Read the model definition and answer for the solid it produces. Units are mm, in the model's axes. Give positions to 0.01 mm unless a question says otherwise; leave off trailing zeros. Order: outer loops, then holes, each group sorted by start corner. A loop starts at its lowest first (then second) coordinate and runs counter-clockwise, first axis right, second up. Notation, with made-up numbers: (22.25, -35.5) - (44.25, -35.5) arc R29 ccw to (44.25, -10.5) - close; hole circle Ø6 at (19.5, -20). An arc over 180 degrees is marked (long way). Use a Markdown table: item, result. Add a question column.
1. A flat-ended cylindrical pin translates along its axis: P1, Ø8.5, axis at x = 24, y = 15, coming from the +Z side. Find the tip coordinate at first contact, or state that the pin passes through.
2. For a pull along Y with two mould halves and no side action, classify faces 1 (the flat face through (109, 0, 5)), 2 (the cylindrical face through (109.1, 170.9, 4.9)), 3 (the flat face through (220, 175, 5)) as released by +Y, released by -Y, zero draft, split by the parting line, or undercut.
3. A cutting plane is placed at A-A on x = 110. Determine the outline of the cut face in (y, z).
4. Consider L1, parallel to Y at x = 24, z = 2.75; L2, parallel to Y at x = 109.5, z = 9.25; L3, parallel to X at y = 189.5, z = 1.75. Determine where each line is inside the solid, lowest interval first.
```python
from build123d import *

# Parameters (mm, degrees)
F0_R     = 7
F1_DEPTH = 10


with BuildPart() as f1:
    # F0 (on Top) → F1 (new body)
    with BuildSketch(Plane.XY):
        with BuildLine():
            ThreePointArc((0, 12), (3.514719, 3.514719), (12, 0))
            Line((12, 0), (208, 0))
            ThreePointArc((208, 0), (216.485281, 3.514719), (220, 12))
            Line((220, 12), (220, 343))
            ThreePointArc((220, 343), (216.485281, 351.485281), (208, 355))
            Line((208, 355), (12, 355))
            ThreePointArc((12, 355), (3.514719, 351.485281), (0, 343))
            Line((0, 343), (0, 12))
        make_face()
        with Locations((24, 15)):
            Circle(F0_R, mode=Mode.SUBTRACT)
        with Locations((196, 15)):
            Circle(F0_R, mode=Mode.SUBTRACT)
        with Locations((110, 163.956369)):
            Circle(F0_R, mode=Mode.SUBTRACT)
        with Locations((24, 188.956369)):
            Circle(F0_R, mode=Mode.SUBTRACT)
        with Locations((196, 188.956369)):
            Circle(F0_R, mode=Mode.SUBTRACT)
        with Locations((110, 337.912739)):
            Circle(F0_R, mode=Mode.SUBTRACT)
    extrude(amount=F1_DEPTH)


solid = f1.part
```
Output values:
| question | item | result |
|---|---|---|
| 1 | P1 | through |
| 2 | face 1 | released by -Y |
| 2 | face 2 | undercut |
| 2 | face 3 | zero draft |
| 3 | outline | (0, 0) - (156.96, 0) - (156.96, 10) - (0, 10) - close; (170.96, 0) - (330.91, 0) - (330.91, 10) - (170.96, 10) - close; (344.91, 0) - (355, 0) - (355, 10) - (344.91, 10) - close |
| 4 | L1 | 0 to 8, 22 to 181.96, 195.96 to 355 |
| 4 | L2 | 0 to 156.97, 170.94 to 330.93, 344.89 to 355 |
| 4 | L3 | 0 to 17.02, 30.98 to 189.02, 202.98 to 220 |
